Read the model definition and answer for the solid it produces. Units are mm, in the model's axes. Face numbers are marked on the shaded views. A direction names the side the tool comes from. Coordinates: 2 decimals unless noted, no trailing zeros. Write each loop counter-clockwise with the first axis right and the second up, starting at its lowest first coordinate (ties: lowest second). Pieces come first, ordered by that corner, then holes. Notation, with made-up numbers: (-16.5, 8.25) - (13.5, 8.25) arc R28 ccw to (13.5, 46.25) - close; hole circle Ø9 at (42, 53). An arc over 180 degrees is marked (long way). Return JSON: item names as keys, results as strings.
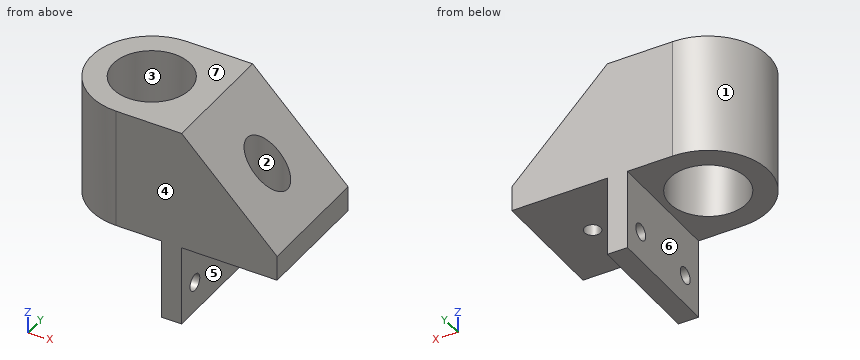
```python
from build123d import *

# Parameters (mm, degrees)
ESBO_O1_R                = 7.65
ESBO_O1_R_2              = 1.6
RESSALTO_EXTRUS_O1_DEPTH = 40
ESBO_O2_W                = 19
ESBO_O2_H                = 20
ESBO_O2_W_2              = 21
ESBO_O2_H_2              = 16
CORTE_EXTRUS_O1_DEPTH    = 67.603303221
ESBO_O3_R                = 1.65
ESBO_O3_W                = 40
ESBO_O3_H                = 6
CORTE_EXTRUS_O2_DEPTH    = 20
CHANFRO2_SIZE            = 20
ESBO_O4_R                = 4
CORTE_EXTRUS_O3_DEPTH    = 19


with BuildPart() as part:
    # Esboço1 → Ressalto-extrusão1 (new body)
    with BuildSketch(Plane.XY):
        with BuildLine():
            Line((0, 0), (-19, 0))
            Line((-19, 0), (-19, 6))
            Line((-19, 6), (-23, 6))
            Line((-23, 6), (-23, 0))
            Line((-23, 0), (-32, 0))
            ThreePointArc((-32, 0), (-44, -12), (-32, -24))
            Line((-32, -24), (-23, -24))
            Line((-23, -24), (-23, -30))
            Line((-23, -30), (-19, -30))
            Line((-19, -30), (-19, -24))
            Line((-19, -24), (0, -24))
            Line((0, -24), (0, 0))
        make_face()
        with Locations((-32, -12)):
            Circle(ESBO_O1_R, mode=Mode.SUBTRACT)
        with Locations((-9, -12)):
            Circle(ESBO_O1_R_2, mode=Mode.SUBTRACT)
    extrude(amount=RESSALTO_EXTRUS_O1_DEPTH)

    # Esboço2 → Corte-extrusão1 (cut, through all)
    with BuildSketch(Plane(origin=(0, 0, 0), x_dir=(1, 0, 0), z_dir=(0, 1, 0))):
        with Locations((-9.5, -30)):
            Rectangle(ESBO_O2_W, ESBO_O2_H)
        with Locations((-33.5, -8)):
            Rectangle(ESBO_O2_W_2, ESBO_O2_H_2)
        with Locations((-9.5, -8)):
            Rectangle(ESBO_O2_W, ESBO_O2_H_2)
    extrude(amount=-CORTE_EXTRUS_O1_DEPTH, mode=Mode.SUBTRACT)

    # Esboço3 → Corte-extrusão2 (cut)
    with BuildSketch(Plane.ZY.offset(23)):
        with Locations((6, -4.5)):
            Circle(ESBO_O3_R)
        with Locations((6, -19.5)):
            Circle(ESBO_O3_R)
        with Locations((20, 3)):
            Rectangle(ESBO_O3_W, ESBO_O3_H)
        with Locations((20, -27)):
            Rectangle(ESBO_O3_W, ESBO_O3_H)
    extrude(amount=-CORTE_EXTRUS_O2_DEPTH, mode=Mode.SUBTRACT)

    # Chanfro2
    # the kernel refuses this chamfer: 20 mm, written as the material it adds along each edge
    with BuildSketch(Plane(origin=(-19, 0, 20), x_dir=(0.9996219169112968, 0, -0.02749587661058649), z_dir=(0, -1, 0))) as chanfro2_piece_1_section:
        Polygon((CHANFRO2_SIZE * 0.999621916911, CHANFRO2_SIZE * 0.0274958766106), (-CHANFRO2_SIZE * 0.0274958766106, CHANFRO2_SIZE * 0.999621916911), (0, 0), align=None)
    chanfro2_piece_1 = extrude(amount=24, mode=Mode.PRIVATE)
    chanfro2_piece_1 = chanfro2_piece_1 - Plane(origin=(-9, -12, 26.656748397), x_dir=(1, 0, 0), z_dir=(0, 0, -1)) * Cylinder(1.6, 128, mode=Mode.PRIVATE)
    chanfro2_piece_1 = split(chanfro2_piece_1, bisect_by=Plane(origin=(0, -11.999999472, 26.656748397), z_dir=(-1, 0, 0)), keep=Keep.TOP, mode=Mode.PRIVATE)
    chanfro2_piece_1 = split(chanfro2_piece_1, bisect_by=Plane(origin=(-12.552402044, -11.999999472, 40), z_dir=(0, 0, -1)), keep=Keep.TOP, mode=Mode.PRIVATE)
    add(chanfro2_piece_1)

    # Esboço4 → Corte-extrusão3 (cut)
    with BuildSketch(Plane.XY.offset(40)):
        with Locations((-9, -12)):
            Circle(ESBO_O4_R)
    extrude(amount=-CORTE_EXTRUS_O3_DEPTH, mode=Mode.SUBTRACT)


solid = part.part
```
(1) A cutting plane is placed at B-B (y = -16.75). Determine the outline of the cut face in (x, z).
Answer:
{"outline": "(-43.02, 16) - (-38, 16) - (-38, 40) - (-43.02, 40) - close; (-26, 16) - (-23, 16) - (-23, 0) - (-19, 0) - (-19, 16) - (0, 16) - (0, 21) - (-19, 40) - (-26, 40) - close"}
(2) Flat-ended cylindrical pins translate along their axes: P1, Ø9, axis at x = -8.5, y = -12.5, coming from the +Z side; P2, Ø3.5, axis at x = -9, y = -12, coming from the +Z side; P3, Ø10.5, axis at x = -28.5, y = -17.5, coming from the -Z side. Find the tip coordinate at first contact, or state that the pin passes through.
Answer:
{"P1": "z = 34", "P2": "z = 21", "P3": "z = 16"}
(3) A cutting plane is placed at C-C (z = 6). Determine the outline of the cut face in (x, y).
Answer:
{"outline": "(-23, -24) - (-19, -24) - (-19, -21.15) - (-23, -21.15) - close; (-23, -17.85) - (-19, -17.85) - (-19, -6.15) - (-23, -6.15) - close; (-23, -2.85) - (-19, -2.85) - (-19, 0) - (-23, 0) - close"}
(4) A cutting plane is placed at D-D (y = -12). Determine the outline of the cut face in (x, z).
Answer:
{"outline": "(-44, 16) - (-39.65, 16) - (-39.65, 40) - (-44, 40) - close; (-24.35, 16) - (-23, 16) - (-23, 0) - (-19, 0) - (-19, 16) - (-10.6, 16) - (-10.6, 21) - (-13, 21) - (-13, 34) - (-19, 40) - (-24.35, 40) - close; (-7.4, 16) - (0, 16) - (0, 21) - (-5, 26) - (-5, 21) - (-7.4, 21) - close"}
(5) Straight lines are drawn through the part: line 1 (Y direction, x = -9, z = 20); line 2 (X direction, y = -12, z = 20.35); line 3 (X direction, y = -12, z = 22). For each, find the intervals that lie inside material, in ascending order. Write a range as from..to.
Answer:
{"line 1": "-24..-13.6, -10.4..0", "line 2": "-44..-39.65, -24.35..-10.6, -7.4..0", "line 3": "-44..-39.65, -24.35..-13, -5..-1"}
(6) Determine the mould class of the marked faces 1, 2, 3 and 4 for opening direction Y: +Y half, -Y half, draft (parallel to the pull), parting line (faces both ways), or undercut.
Answer:
{"face 1": "parting line", "face 2": "undercut", "face 3": "undercut", "face 4": "-Y half"}
(7) Which of the six approach directions +Z, -Z, +X, -X, +Y, -Y give full straight-line access (tool end or side, diameter ignored) to the marked faces 5, 6 and 7?
Answer:
{"face 5": "-Z, +X, +Y, -Y", "face 6": "-Z, -X, +Y, -Y", "face 7": "+Z, +X, -X, +Y, -Y"}
(8) A cutting plane is placed at A-A (x = -9). Determine the outline of the cut face in (y, z), and give its area (3 significant figures).
Answer:
{"outline": "(-24, 16) - (-13.6, 16) - (-13.6, 21) - (-16, 21) - (-16, 30) - (-24, 30) - close; (-10.4, 16) - (0, 16) - (0, 30) - (-8, 30) - (-8, 21) - (-10.4, 21) - close", "area": "248 mm²"}
